from build123d import *

# Parameters (mm, degrees)
RESSALTO_EXTRUS_O1_DEPTH = 50
ESBO_O2_R                = 5.15
CORTE_EXTRUS_O1_DEPTH    = 3.5
ESBO_O3_R                = 5.15
CORTE_EXTRUS_O2_DEPTH    = 3.5
RESSALTO_EXTRUS_O2_DEPTH = 2.5
ESBO_O5_R                = 2
CORTE_EXTRUS_O3_DEPTH    = 10
ESBO_O6_R                = 2
CORTE_EXTRUS_O4_DEPTH    = 10


with BuildPart() as part:
    # Esboço1 → Ressalto-extrusão1 (new body)
    with BuildSketch(Plane.XY):
        Polygon((0, 0), (35, 0), (35, 4), (-4, 4), (-4, -20), (0, -20), align=None)
    extrude(amount=RESSALTO_EXTRUS_O1_DEPTH)

    # Esboço2 → Corte-extrusão1 (cut)
    with BuildSketch(Plane(origin=(0, 0, 0), x_dir=(0, 0, -1), z_dir=(1, 0, 0))):
        with Locations((-42, -12)):
            Circle(ESBO_O2_R)
        with Locations((-12, -12)):
            Circle(ESBO_O2_R)
    extrude(amount=-CORTE_EXTRUS_O1_DEPTH, mode=Mode.SUBTRACT)

    # Esboço3 → Corte-extrusão2 (cut)
    with BuildSketch(Plane.XZ):
        with Locations((12, 42)):
            Circle(ESBO_O3_R)
        with Locations((12, 12)):
            Circle(ESBO_O3_R)
    extrude(amount=-CORTE_EXTRUS_O2_DEPTH, mode=Mode.SUBTRACT)

    # Esboço4 → Ressalto-extrusão2 (add)
    with BuildSketch(Plane.XY.offset(50)):
        Polygon((0, -20), (20, 0), (35, 0), (35, 4), (-4, 4), (-4, -20), align=None)
    extrude(amount=RESSALTO_EXTRUS_O2_DEPTH)

    # Esboço5 → Corte-extrusão3 (cut)
    with BuildSketch(Plane.XZ.offset(-3.5)):
        with Locations((12, 42)):
            Circle(ESBO_O5_R)
        with Locations((12, 12)):
            Circle(ESBO_O5_R)
    extrude(amount=-CORTE_EXTRUS_O3_DEPTH, mode=Mode.SUBTRACT)

    # Esboço6 → Corte-extrusão4 (cut)
    with BuildSketch(Plane(origin=(-3.5, 0, 0), x_dir=(0, 0, -1), z_dir=(1, 0, 0))):
        with Locations((-42, -12)):
            Circle(ESBO_O6_R)
        with Locations((-12, -12)):
            Circle(ESBO_O6_R)
    extrude(amount=-CORTE_EXTRUS_O4_DEPTH, mode=Mode.SUBTRACT)


solid = part.part
Model file for the job. Use its own axes, mm. A direction names the side the tool comes from. Give positions to 0.01 mm unless a question says otherwise; leave off trailing zeros. Write each loop counter-clockwise with the first axis right and the second up, starting at its lowest first coordinate (ties: lowest second). Pieces come first, ordered by that corner, then holes. Notation, with made-up numbers: (67.25, 78) -> (72.25, 78) arc R23 cw to (72.25, 98) -> close; hole circle Ø1 at (86, 78.5). An arc over 180 degrees is marked (long way). Write item = value, one per line.
(1) Slice it at B-B, the plane x = 12. Give the cut face in (y, z), then the cut area to 3 significant figures.
Determined:
outline = (-8, 50) -> (0, 50) -> (0, 47.15) -> (3.5, 47.15) -> (3.5, 44) -> (4, 44) -> (4, 52.5) -> (-8, 52.5) -> close; (0, 0) -> (4, 0) -> (4, 10) -> (3.5, 10) -> (3.5, 6.85) -> (0, 6.85) -> close; (0, 17.15) -> (3.5, 17.15) -> (3.5, 14) -> (4, 14) -> (4, 40) -> (3.5, 40) -> (3.5, 36.85) -> (0, 36.85) -> close
area = 154 mm2
(2) Tool access for faces 4 (the face through (14.2, 3.5, 42.1)), 5 (the face through (16, 4, 26)), 6 (the face through (-3.5, -11.9, 9.8)), 7 (the face through (0, -10, 25)): list every direction of +Z, -Z, +X, -X, +Y, -Y with a clear straight run to the whole face (end or side of a thin tool).
Determined:
face_4 = -Y
face_5 = +Z, -Z, +X, -X, +Y
face_6 = +X
face_7 = -Z, +X, -Y
(3) Slice it at D-D, the plane y = -3.25. Give the cut face in (x, z).
Determined:
outline = (-4, 0) -> (0, 0) -> (0, 50) -> (16.75, 50) -> (16.75, 52.5) -> (-4, 52.5) -> close
(4) Flat gauge pins, fed straight in: P1, Ø10, axis at x = 8, y = -12, coming from the -Z side; P2, Ø6, axis at x = 16.5, z = 10.5, coming from the -Y side; P3, Ø13.5, axis at y = -12, z = 12, coming from the +X side; P4, Ø9.5, axis at x = 12, z = 12, coming from the +Y side. Where does each tip first touch, or does it go through?
Determined:
P1 = 50
P2 = 0
P3 = 0
P4 = 4
(5) Mould opens along Y. For faces 1 (the face through (17, 0, 26)), 2 (the face through (35, 2, 26)), 3 (the face through (-1.726, -17.028, 13.116)) say: released by +Y, released by -Y, zero draft, split by the parting line, or undercut.
Determined:
face_1 = released by -Y
face_2 = zero draft
face_3 = undercut
(6) Slice it at C-C, the plane z = 21. Give the cut face in (x, y).
Determined:
outline = (-4, -20) -> (0, -20) -> (0, 0) -> (35, 0) -> (35, 4) -> (-4, 4) -> close
(7) Slice it at A-A, the plane z = 42. Give the cut face in (x, y), then the cut area to 3 significant figures.
Determined:
outline = (-4, -20) -> (0, -20) -> (0, -17.15) -> (-3.5, -17.15) -> (-3.5, -14) -> (-4, -14) -> close; (-4, -10) -> (-3.5, -10) -> (-3.5, -6.85) -> (0, -6.85) -> (0, 0) -> (6.85, 0) -> (6.85, 3.5) -> (10, 3.5) -> (10, 4) -> (-4, 4) -> close; (14, 3.5) -> (17.15, 3.5) -> (17.15, 0) -> (35, 0) -> (35, 4) -> (14, 4) -> close
area = 160 mm2
(8) Probe line 1 along Y through (x, z) = (-2.05, 12); line 2 along Y through (x, z) = (0.5, 45.5); line 3 along Z through (x, y) = (1.5, -7.25). List the from-to ranges inside material, lowest first.
Determined:
line_1 = -20 to -17.15, -6.85 to 4
line_2 = 0 to 4
line_3 = 50 to 52.5
